```python
from build123d import *

# Parameters (mm, degrees)
SKETCH1_W           = 50.8
SKETCH1_H           = 50.8
BOSS_EXTRUDE1_DEPTH = 215.9
SHELL1_T            = -3.175
SKETCH2_R           = 14.3129
CUT_EXTRUDE1_DEPTH  = 224.245627057
SKETCH3_R           = 2.38125
CUT_EXTRUDE2_DEPTH  = 224.245627057
SKETCH4_R           = 2.38125
CUT_EXTRUDE3_DEPTH  = 224.245627057
SKETCH5_R           = 2.38125
CUT_EXTRUDE4_DEPTH  = 224.245627057


with BuildPart() as part:
    # Sketch1 → Boss-Extrude1 (new body)
    with BuildSketch(Plane(origin=(0, 0, 0), x_dir=(1, 0, 0), z_dir=(0, 1, 0))):
        Rectangle(SKETCH1_W, SKETCH1_H)
    extrude(amount=BOSS_EXTRUDE1_DEPTH)

    # Shell1
    shell1_openings = [part.faces().sort_by_distance(p)[0] for p in [
        (0, 215.9, 0),
        (0, 0, 0),
    ]]
    offset(amount=SHELL1_T, openings=shell1_openings, kind=Kind.INTERSECTION)

    # Sketch2 → Cut-Extrude1 (cut, through all)
    with BuildSketch(Plane(origin=(25.4, 0, 0), x_dir=(0, 0, -1), z_dir=(1, 0, 0))):
        with Locations((0, 31.75)):
            Circle(SKETCH2_R)
    extrude(amount=-CUT_EXTRUDE1_DEPTH, mode=Mode.SUBTRACT)

    # Sketch3 → Cut-Extrude2 (cut, through all)
    with BuildSketch(Plane(origin=(25.4, 0, 0), x_dir=(0, 0, -1), z_dir=(1, 0, 0))):
        with Locations((-11.90625, 52.372229928)):
            Circle(SKETCH3_R)
        with Locations((11.90625, 52.372229928)):
            Circle(SKETCH3_R)
        with Locations((-11.90625, 11.127770072)):
            Circle(SKETCH3_R)
        with Locations((11.90625, 11.127770072)):
            Circle(SKETCH3_R)
    extrude(amount=-CUT_EXTRUDE2_DEPTH, mode=Mode.SUBTRACT)

    # Sketch4 → Cut-Extrude3 (cut, through all)
    with BuildSketch(Plane(origin=(25.4, 0, 0), x_dir=(0, 0, -1), z_dir=(1, 0, 0))):
        with Locations((-12.7, 203.2)):
            Circle(SKETCH4_R)
        with Locations((12.7, 203.2)):
            Circle(SKETCH4_R)
        with Locations((12.7, 177.8)):
            Circle(SKETCH4_R)
        with Locations((-12.7, 177.8)):
            Circle(SKETCH4_R)
    extrude(amount=-CUT_EXTRUDE3_DEPTH, mode=Mode.SUBTRACT)

    # Sketch5 → Cut-Extrude4 (cut, through all)
    with BuildSketch(Plane.XY.offset(25.4)):
        with Locations((-12.7, 203.2)):
            Circle(SKETCH5_R)
        with Locations((12.7, 203.2)):
            Circle(SKETCH5_R)
        with Locations((12.7, 177.8)):
            Circle(SKETCH5_R)
        with Locations((-12.7, 177.8)):
            Circle(SKETCH5_R)
    extrude(amount=-CUT_EXTRUDE4_DEPTH, mode=Mode.SUBTRACT)


solid = part.part
```
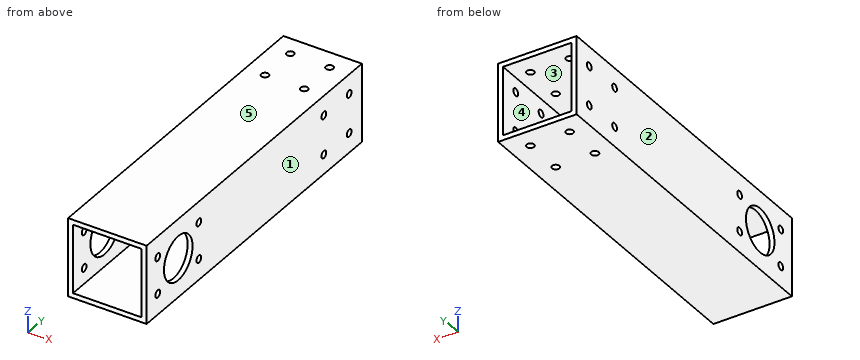
The listing builds one solid part. Answer for the finished solid, in the listing's coordinates (mm). Face numbers are marked on the shaded views. A direction names the side the tool comes from. Coordinates: 2 decimals unless noted, no trailing zeros. Write each loop counter-clockwise with the first axis right and the second up, starting at its lowest first coordinate (ties: lowest second). Pieces come first, ordered by that corner, then holes.
Q1. Given P1, Ø4, axis at y = 177.8, z = -12.7, coming from the +X side, flat-ended and moving along its own axis, determine where the tip first touches the part or whether it passes through.
Returned:
P1: passes through
Q2. Section C-C, the plane x = -2 is taken. Write down the section's boundary in (y, z) (3 decimals).
Returned:
outline: (0, -25.4) - (215.9, -25.4) - (215.9, -22.225) - (0, -22.225) - close; (0, 22.225) - (215.9, 22.225) - (215.9, 25.4) - (0, 25.4) - close
Q3. Section A-A, the plane z = 20 is taken. Write down the section's boundary in (x, y) (3 decimals), then the cut area to 3 significant figures.
Returned:
outline: (-25.4, 0) - (-22.225, 0) - (-22.225, 215.9) - (-25.4, 215.9) - close; (22.225, 0) - (25.4, 0) - (25.4, 215.9) - (22.225, 215.9) - close
area: 1,370 mm2
Q4. The mould has two halves that part along X. Classify the marked faces 1, 2 and 3: released by +X, released by -X, zero draft, split by the parting line, or undercut.
Returned:
face 1: released by +X
face 2: released by -X
face 3: undercut
Q5. Find the intervals of material crossed by line 1 along Z through (x, y) = (-24.6, 203.2); line 2 along X through (y, z) = (203, 24); line 3 along X through (y, z) = (146.5, -18) (3 decimals), in increasing order.
Returned:
line 1: z = -25.4 to -15.08, -10.32 to 10.32, 15.08 to 25.4
line 2: x = -25.4 to -15.07, -10.33 to 10.33, 15.07 to 25.4
line 3: x = -25.4 to -22.225, 22.225 to 25.4
Q6. Section D-D, the plane y = 136.5 is taken. Write down the section's boundary in (x, z) (3 decimals), then the cut area to 3 significant figures.
Returned:
outline: (-25.4, -25.4) - (25.4, -25.4) - (25.4, 25.4) - (-25.4, 25.4) - close; hole (-22.225, -22.225) - (22.225, -22.225) - (22.225, 22.225) - (-22.225, 22.225) - close
area: 605 mm2
Q7. Which of the six approach directions +Z, -Z, +X, -X, +Y, -Y give full straight-line access (tool end or side, diameter ignored) to the marked faces 4 and 5?
Returned:
face 4: +Y, -Y
face 5: +Z, +X, -X, +Y, -Y
Q8. Section B-B, the plane x = 12.7 is taken. Write down the section's boundary in (y, z) (3 decimals).
Returned:
outline: (0, -25.4) - (175.419, -25.4) - (175.419, -22.225) - (0, -22.225) - close; (0, 22.225) - (175.419, 22.225) - (175.419, 25.4) - (0, 25.4) - close; (180.181, -25.4) - (200.819, -25.4) - (200.819, -22.225) - (180.181, -22.225) - close; (180.181, 22.225) - (200.819, 22.225) - (200.819, 25.4) - (180.181, 25.4) - close; (205.581, -25.4) - (215.9, -25.4) - (215.9, -22.225) - (205.581, -22.225) - close; (205.581, 22.225) - (215.9, 22.225) - (215.9, 25.4) - (205.581, 25.4) - close
